```python
from build123d import *

# Parameters (mm, degrees)
SKETCH1_R           = 49.53
SKETCH1_R_2         = 40.64
BOSS_EXTRUDE1_DEPTH = 12.7
BOSS_EXTRUDE2_START = -12.7
BOSS_EXTRUDE2_DEPTH = 25.4
SKETCH3_R           = 9.525
CUT_EXTRUDE1_DEPTH  = 88.729988813
CIRPATTERN1_COUNT   = 4


# Read off the part's stored shape, not the designer's step: Boss-Extrude2
with BuildPart() as part:
    # Sketch1 → Boss-Extrude1 (new, symmetric)
    with BuildSketch(Plane(origin=(0, 0, 0), x_dir=(1, 0, 0), z_dir=(0, 1, 0))):
        with Locations(Location((0, 0, 0), (0, 0, 270))):
            Circle(SKETCH1_R)
        with Locations(Location((0, 0, 0), (0, 0, 270))):
            Circle(SKETCH1_R_2, mode=Mode.SUBTRACT)
    extrude(amount=BOSS_EXTRUDE1_DEPTH, both=True)

    # Boss-Extrude2 outline → Boss-Extrude2 (add)
    with BuildSketch(Plane(origin=(0, 0, 0), x_dir=(1, 0, 0), z_dir=(0, 1, 0)).offset(BOSS_EXTRUDE2_START)):
        with BuildLine():
            ThreePointArc((-14.773428494, 37.859680539), (-25.835391963, 31.371039545), (-34.324632471, 21.758428384))
            Line((-34.324632471, 21.758428384), (-14.773428494, 21.758428384))
            Line((-14.773428494, 21.758428384), (-14.773428494, 37.859680539))
        make_face()
        with BuildLine():
            Line((-21.758428494, -14.773428384), (-37.859680582, -14.773428384))
            ThreePointArc((-37.859680582, -14.773428384), (-31.371039624, -25.835391867), (-21.758428494, -34.324632401))
            Line((-21.758428494, -34.324632401), (-21.758428494, -14.773428384))
        make_face()
        with BuildLine():
            ThreePointArc((37.859680582, 14.773428384), (31.371039624, 25.835391867), (21.758428494, 34.324632401))
            Line((21.758428494, 34.324632401), (21.758428494, 14.773428384))
            Line((21.758428494, 14.773428384), (37.859680582, 14.773428384))
        make_face()
        with BuildLine():
            Line((14.773428494, -21.758428384), (14.773428494, -37.859680539))
            ThreePointArc((14.773428494, -37.859680539), (25.835391963, -31.371039545), (34.324632471, -21.758428384))
            Line((34.324632471, -21.758428384), (14.773428494, -21.758428384))
        make_face()
    extrude(amount=BOSS_EXTRUDE2_DEPTH)

    # Sketch3 → Cut-Extrude1 (cut, through all)
    with BuildSketch(Plane(origin=(-21.758428494, 0, 0), x_dir=(0, 0, -1), z_dir=(1, 0, 0))):
        with Locations((-24.549030393, 0)):
            Circle(SKETCH3_R)
    cut_extrude1 = extrude(amount=-CUT_EXTRUDE1_DEPTH, mode=Mode.SUBTRACT)

    # CirPattern1: Cut-Extrude1 ×4 about axis
    cirpattern1_axis = Axis((0, 0, 0), (0, 1, 0))
    for i in range(1, CIRPATTERN1_COUNT):
        add(cut_extrude1.rotate(cirpattern1_axis, i * 360 / CIRPATTERN1_COUNT), mode=Mode.SUBTRACT)


solid = part.part
```
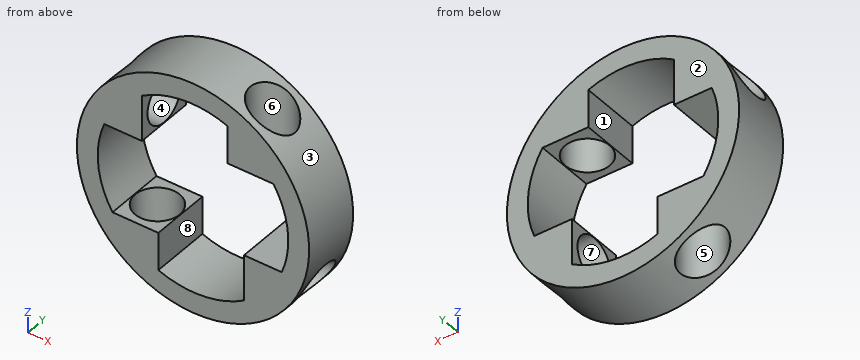
Geometry check sheet. Reference: the model listing, model coordinates, mm. Face numbers are marked on the shaded views. A direction names the side the tool comes from. Give positions to 0.01 mm unless a question says otherwise; leave off trailing zeros. Order: outer loops, then holes, each group sorted by start corner. A loop starts at its lowest first (then second) coordinate and runs counter-clockwise, first axis right, second up. Notation, with made-up numbers: (-38, 81) - (11, 81) arc R4 ccw to (11, 86) - close; hole circle Ø8 at (-39, 36). An arc over 180 degrees is marked (long way). Write item = value, one per line. Start each with the question number.
1) Section check B-B (x = 0). Enter the section's corners in (y, z), then the cut area to 3 significant figures.
2) Access from +Z, -Z, +X, -X, +Y, -Y to the whole of each face (thin tool, end or side, straight path). Record for the marked faces 4, 5, 6, 7 and 8.
3) Section check A-A (z = -32.5). Enter the section's corners in (x, y) (3 decimals), then the cut area to 3 significant figures.
4) Draft check along Z on the marked faces 1, 2 and 3. Enter one of: released by +Z, released by -Z, zero draft, split by the parting line, or undercut.
5) Section check D-D (z = 0). Enter the section's corners in (x, y), then the cut area to 3 significant figures.
6) Section check C-C (y = -1.25). Enter the section's corners in (x, z).
7) Gauge pin test, flat ends, axial feed: pin 1 Ø15 at (x, y) = (24.55, 0) entering from -Z; pin 2 Ø10 at (y, z) = (-3.5, -29) entering from -X; pin 3 Ø2 at (x, y) = (-1.5, 9.5) entering from +Z. Record the tip position at first contact, or that the pin passes through.
8) Scan lines: L1, parallel to X at y = -0.5, z = -1; L2, parallel to X at y = 7.5, z = 8.5; L3, parallel to Y at x = 18, z = 33. Record each from-to range of solid material in increasing order.
Geometry check:
q1.outline = (-12.7, -49.53) - (12.7, -49.53) - (12.7, -40.64) - (-12.7, -40.64) - close; (-12.7, 40.64) - (12.7, 40.64) - (12.7, 49.53) - (-12.7, 49.53) - close
q1.area = 452 mm2
q2.face_4 = -X
q2.face_5 = -Z
q2.face_6 = +Z
q2.face_7 = +X
q2.face_8 = +Y, -Y
q3.outline = (-37.376, -12.7) - (-14.773, -12.7) - (-14.773, 12.7) - (-37.376, 12.7) - close; (21.758, -12.7) - (37.376, -12.7) - (37.376, -5.245) - (21.758, -5.245) - close; (21.758, 5.245) - (37.376, 5.245) - (37.376, 12.7) - (21.758, 12.7) - close; hole circle Ø19.05 at (-24.549, 0)
q3.area = 522 mm2
q4.face_1 = undercut
q4.face_2 = zero draft
q4.face_3 = split by the parting line
q5.outline = (-49.53, -12.7) - (-40.64, -12.7) - (-40.64, 12.7) - (-49.53, 12.7) - close; (40.64, -12.7) - (49.53, -12.7) - (49.53, 12.7) - (40.64, 12.7) - close
q5.area = 452 mm2
q6.outline = (-47.17, 15.11) arc R49.53 ccw to (-33.99, -36.02) - (-33.99, -21.76) - (-34.32, -21.76) arc R40.64 cw to (-37.86, 14.77) - (-21.76, 14.77) - (-21.76, 15.11) - close; (-36.02, 33.99) - (-21.76, 33.99) - (-21.76, 34.32) arc R40.64 cw to (14.77, 37.86) - (14.77, 21.76) - (15.11, 21.76) - (15.11, 47.17) arc R49.53 ccw to start; (-15.11, -47.17) arc R49.53 ccw to (36.02, -33.99) - (21.76, -33.99) - (21.76, -34.32) arc R40.64 cw to (-14.77, -37.86) - (-14.77, -21.76) - (-15.11, -21.76) - close; (21.76, -15.11) - (47.17, -15.11) arc R49.53 ccw to (33.99, 36.02) - (33.99, 21.76) - (34.32, 21.76) arc R40.64 cw to (37.86, -14.77) - (21.76, -14.77) - close
q7.pin_1 = -46.5
q7.pin_2 = -43.33
q7.pin_3 = 49.53
q8.L1 = -49.52 to -40.63, 40.63 to 49.52
q8.L2 = -48.8 to -39.74, 39.74 to 48.8
q8.L3 = -12.7 to -6.92, 6.92 to 12.7
